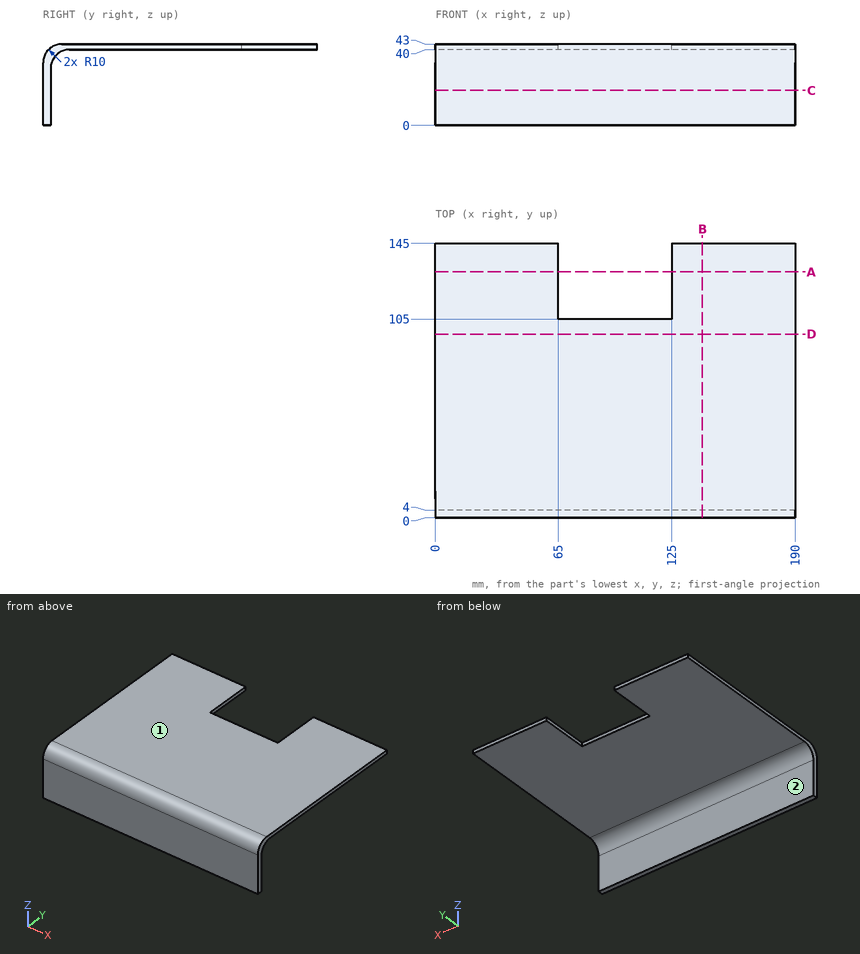
Drawing for the job (mm, zero at the part's lowest x, y, z). A direction names the side the tool comes from. Round coordinates to 2 decimals unless told otherwise and drop trailing zeros. Order: outer loops, then holes, each group sorted by start corner. A loop starts at its lowest first (then second) coordinate and runs counter-clockwise, first axis right, second up. Notation, with made-up numbers: (-15, 3) -> (26, 3) arc R21 ccw to (26, 15) -> close; hole circle Ø1 at (41.25, 16.25). An arc over 180 degrees is marked (long way). Write item = value, one per line. Start each with the question number.
(1) Cut at D-D, the plane y = 97. List the corners of the cut face in (x, z).
(2) Cut at C-C, the plane z = 18.5. List the corners of the cut face in (x, y), then the cut area to 3 significant figures.
(3) Cut at A-A, the plane y = 130. List the corners of the cut face in (x, z), then the cut area to 3 significant figures.
(4) Cut at B-B, the plane x = 141. List the corners of the cut face in (y, z), then the cut area to 3 significant figures.
(5) Which spindle directions (+Z, -Z, +X, -X, +Y, -Y) get a long thin tool onto all of the face, cutting with end or side? Do the marked faces 1 and 2. Say none if no direction does.
(6) Probe line 1 (Y direction, x = 162, z = 25.5); line 2 (Z direction, x = 53, y = 68); line 3 (Y direction, x = 159, z = 32). List the from-to ranges inside material, lowest first. Write a range as [from, to].
(7) Pin check, flat tips, straight feed: P1, Ø0.9, axis at x = 105, z = 42, coming from the +Y side; P2, Ø5, axis at x = 133.5, y = 42.5, coming from the -Z side; P3, Ø6, axis at x = 66, z = 25.5, coming from the +Y side; P4, Ø8, axis at y = 62, z = 34.5, coming from the +X side. Stop position of each tip, or through.
Model answer:
q1.outline = (0, 40) -> (190, 40) -> (190, 43) -> (0, 43) -> close
q2.outline = (0, 0) -> (190, 0) -> (190, 4) -> (0, 4) -> close
q2.area = 760 mm2
q3.outline = (0, 40) -> (65, 40) -> (65, 43) -> (0, 43) -> close; (125, 40) -> (190, 40) -> (190, 43) -> (125, 43) -> close
q3.area = 390 mm2
q4.outline = (0, 0) -> (4, 0) -> (4, 30) arc R10 cw to (14, 40) -> (145, 40) -> (145, 43) -> (10, 43) arc R10 ccw to (0, 33) -> close
q4.area = 595 mm2
q5.face_1 = +Z, +X, -X, +Y, -Y
q5.face_2 = -Z, +X, -X, +Y
q6.line_1 = [0, 4]
q6.line_2 = [40, 43]
q6.line_3 = [0, 4.2]
q7.P1 = 105
q7.P2 = 40
q7.P3 = 4
q7.P4 = through
